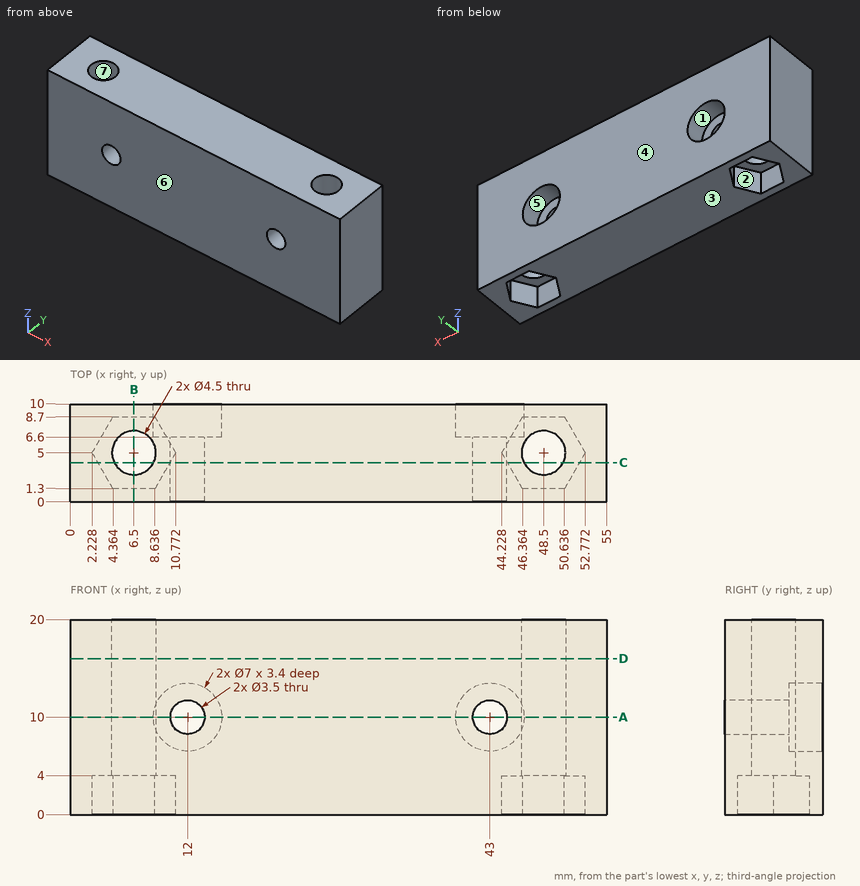
The figure shows three views and two pictorial views of one solid part (mm, origin at its lowest corner). Answer the questions. A direction names the side the tool comes from. Give positions to 0.01 mm unless a question says otherwise; leave off trailing zeros. Write each loop counter-clockwise with the first axis right and the second up, starting at its lowest first coordinate (ties: lowest second). Pieces come first, ordered by that corner, then holes. Notation, with made-up numbers: (47, -37.75) -> (95, -37.75) arc R13 cw to (95, -16.75) -> close; hole circle Ø1 at (0, 49.25). An arc over 180 degrees is marked (long way). Use one line per item in the form item = value.
1) Straight lines are drawn through the part: probe 1 along X at (y, z) = (1.75, 10); probe 2 along Y at (x, z) = (48.5, 9.5); probe 3 along X at (y, z) = (5, 2). For each, find the intervals that lie inside material, in ascending order.
Result:
probe_1 = 0 to 10.25, 13.75 to 41.25, 44.75 to 55
probe_2 = 0 to 2.75, 7.25 to 10
probe_3 = 0 to 2.23, 10.77 to 44.23, 52.77 to 55
2) Section D-D on z = 16 is taken. Write down the section's boundary in (x, y), plus the area to 3 significant figures.
Result:
outline = (0, 0) -> (55, 0) -> (55, 10) -> (0, 10) -> close; hole circle Ø4.5 at (6.5, 5); hole circle Ø4.5 at (48.5, 5)
area = 518 mm²
3) Section A-A on z = 10 is taken. Write down the section's boundary in (x, y).
Result:
outline = (0, 0) -> (10.25, 0) -> (10.25, 6.6) -> (8.5, 6.6) -> (8.5, 10) -> (0, 10) -> close; (13.75, 0) -> (41.25, 0) -> (41.25, 6.6) -> (39.5, 6.6) -> (39.5, 10) -> (15.5, 10) -> (15.5, 6.6) -> (13.75, 6.6) -> close; (44.75, 0) -> (55, 0) -> (55, 10) -> (46.5, 10) -> (46.5, 6.6) -> (44.75, 6.6) -> close; hole circle Ø4.5 at (6.5, 5); hole circle Ø4.5 at (48.5, 5)
4) Section C-C on y = 4 is taken. Count the separate pieces of the cut face and the enclosed holes in it.
Result:
separate_pieces = 3
enclosed_holes = 2
5) Section B-B on x = 6.5 is taken. Write down the section's boundary in (y, z).
Result:
outline = (0, 0) -> (1.3, 0) -> (1.3, 4) -> (2.75, 4) -> (2.75, 20) -> (0, 20) -> close; (7.25, 4) -> (8.7, 4) -> (8.7, 0) -> (10, 0) -> (10, 20) -> (7.25, 20) -> close
6) A tool of negligible diameter and unlimited length cuts with its end or side. For the marked faces 1, 2 and 3, from which of +Z, -Z, +X, -X, +Y, -Y can it reach the whole face along a straight path? Write none if from no direction.
Result:
face_1 = +Y
face_2 = -Z
face_3 = -Z, +X, -X, +Y, -Y
7) For a pull along Y with two mould halves and no side action, classify the marked faces 4, 5, 6 and 7 as +Y half, -Y half, draft (parallel to the pull), parting line (faces both ways), or undercut.
Result:
face_4 = +Y half
face_5 = draft
face_6 = -Y half
face_7 = undercut
8) Each of these flat-tipped pins is pushed along its axis until it touches: P1, Ø2, axis at y = 2.5, z = 15, coming from the -X side; P2, Ø3.5, axis at x = 48, y = 5.5, coming from the -Z side; P3, Ø2.5, axis at x = 48.5, y = 5, coming from the +Z side; P4, Ø2, axis at x = 12, z = 11, coming from the +Y side. Where does it stop, or does it pass through?
Result:
P1 = 0
P2 = 4
P3 = through
P4 = 6.6
